Check sheet for the modelled part. Datum: model origin and axes. Units: mm. Face numbers are marked on the shaded views. Give positions to 0.01 mm unless a question says otherwise; leave off trailing zeros. Loops run counter-clockwise (first coordinate to the right, second up) from the corner with the lowest first, then second, coordinate; pieces in that order, holes last. Notation, with made-up numbers: M -20,19 L -11,19 A26 cw -11,33 Z; hole C -12.75,53 d2. An arc over 180 degrees is marked long. Use one line per item in the form item = value.
from build123d import *

# Parameters (mm, degrees)
SCHIZZO1_R                   = 3.375
ESTRUSIONE_ESTRUSIONE1_DEPTH = 1.35
SCHIZZO2_R                   = 3.375
ESTRUSIONE_ESTRUSIONE2_DEPTH = 2
SCHIZZO3_R                   = 2.25
TAGLIO_ESTRUSIONE1_DEPTH     = 2
SCHIZZO4_R                   = 1
TAGLIO_ESTRUSIONE2_DEPTH     = 17.47393775


with BuildPart() as part:
    # Schizzo1 → Estrusione-Estrusione1 (new body)
    with BuildSketch(Plane(origin=(0, 0, 0), x_dir=(1, 0, 0), z_dir=(0, 1, 0))):
        Circle(SCHIZZO1_R)
        with BuildLine():
            Line((-2.090005981, 2.65), (-14.5, 1.5))
            ThreePointArc((-14.5, 1.5), (-16, 0), (-14.5, -1.5))
            Line((-14.5, -1.5), (-2.090005981, -2.65))
            Line((-2.090005981, -2.65), (-2.090005981, 2.65))
        make_face()
        with BuildLine():
            Line((2.090005981, 2.65), (2.090005981, -2.65))
            Line((2.090005981, -2.65), (14.5, -1.5))
            ThreePointArc((14.5, -1.5), (16, 0), (14.5, 1.5))
            Line((14.5, 1.5), (2.090005981, 2.65))
        make_face()
    extrude(amount=ESTRUSIONE_ESTRUSIONE1_DEPTH)

    # Schizzo2 → Estrusione-Estrusione2 (add)
    with BuildSketch(Plane(origin=(0, 1.35, 0), x_dir=(1, 0, 0), z_dir=(0, 1, 0))):
        with Locations(Location((0, 0, 0), (0, 0, 128.262191128))):
            Circle(SCHIZZO2_R)
    extrude(amount=ESTRUSIONE_ESTRUSIONE2_DEPTH)

    # Schizzo3 → Taglio-Estrusione1 (cut)
    with BuildSketch(Plane(origin=(0, 3.35, 0), x_dir=(1, 0, 0), z_dir=(0, 1, 0))):
        with Locations(Location((0, 0, 0), (0, 0, 270))):
            Circle(SCHIZZO3_R)
    extrude(amount=-TAGLIO_ESTRUSIONE1_DEPTH, mode=Mode.SUBTRACT)

    # Schizzo4 → Taglio-Estrusione2 (cut, through all)
    with BuildSketch(Plane(origin=(0, 1.35, 0), x_dir=(1, 0, 0), z_dir=(0, 1, 0))):
        with Locations(Location((0, 0, 0), (0, 0, 270))):
            Circle(SCHIZZO4_R)
    extrude(amount=-TAGLIO_ESTRUSIONE2_DEPTH, mode=Mode.SUBTRACT)


solid = part.part
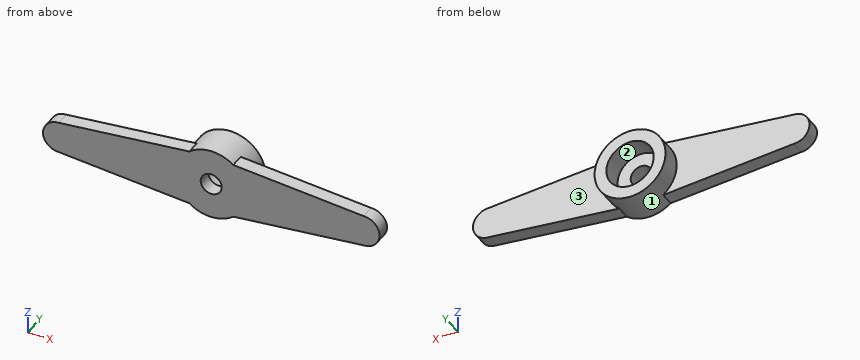
1) Section check C-C (x = 0). Record the cut outline in (y, z) (3 decimals).
Evaluation:
outline = M 0,-3.375 L 3.35,-3.375 L 3.35,-2.25 L 1.35,-2.25 L 1.35,-1 L 0,-1 Z; M 0,1 L 1.35,1 L 1.35,2.25 L 3.35,2.25 L 3.35,3.375 L 0,3.375 Z
2) Release check for a two-part mould opening along X. For the marked faces 1, 2 and 3 record: pulls with the +X half, pulls with the -X half, needs draft (parallel to the pull), parting line crosses it, or undercut.
Evaluation:
face_1 = parting line crosses it
face_2 = undercut
face_3 = needs draft
3) Section check B-B (z = 0). Record the cut outline in (x, y) (3 decimals).
Evaluation:
outline = M -16,0 L -1,0 L -1,1.35 L -2.25,1.35 L -2.25,3.35 L -3.375,3.35 L -3.375,1.35 L -16,1.35 Z; M 1,0 L 16,0 L 16,1.35 L 3.375,1.35 L 3.375,3.35 L 2.25,3.35 L 2.25,1.35 L 1,1.35 Z
4) Scan lines: line 1 (X direction, y = 2.9, z = 0) (3 decimals); line 2 (X direction, y = 0.8, z = 0); line 3 (Y direction, x = -2, z = 0.25). Record each from-to range of solid material in increasing order.
Evaluation:
line_1 = -3.375 to -2.25, 2.25 to 3.375
line_2 = -16 to -1, 1 to 16
line_3 = 0 to 1.35
5) Depth check by flat-ended pin: pin 1 Ø2 at (x, z) = (0.5, 0.5) entering from +Y; pin 2 Ø1.2 at (x, z) = (0, 0) entering from -Y; pin 3 Ø1 at (x, y) = (-1, 2) entering from -Z; pin 4 Ø2 at (x, y) = (-9.5, 1.5) entering from +Z. Enter the tip coordinate at first touch or a pass-through.
Evaluation:
pin_1 = 1.35
pin_2 = through
pin_3 = -3.34
pin_4 = 2.05
6) Section check D-D (y = 2.05). Record the cut outline in (x, z) (3 decimals), then the cut area to 3 significant figures.
Evaluation:
outline = C 0,0 d6.75; hole C 0,0 d4.5
area = 19.9 mm^2
7) Section check A-A (y = 0.75). Record the cut outline in (x, z) (3 decimals), then the cut area to 3 significant figures.
Evaluation:
outline = M -14.5,-1.5 L -2.09,-2.65 A3.375 ccw 2.09,-2.65 L 14.5,-1.5 A1.5 ccw 14.5,1.5 L 2.09,2.65 A3.375 ccw -2.09,2.65 L -14.5,1.5 A1.5 ccw Z; hole C 0,0 d2
area = 133 mm^2
